Build history of the part. All positions in model axes, mm. Face numbers are marked on the shaded views. A direction names the side the tool comes from. Round coordinates to 2 decimals unless told otherwise and drop trailing zeros. Write each loop counter-clockwise with the first axis right and the second up, starting at its lowest first coordinate (ties: lowest second). Pieces come first, ordered by that corner, then holes.
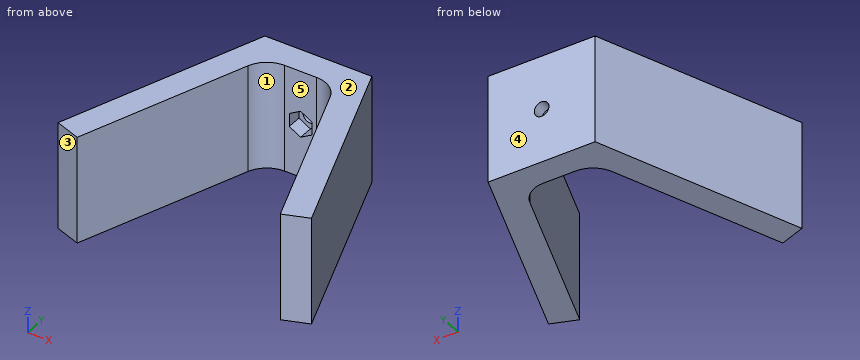
from build123d import *

# Parameters (mm, degrees)
F1_DEPTH = 40
F3_R     = 2.75
F4_DEPTH = 10
F5_R     = 2.75
F6_DEPTH = 5.5
F7_R     = 10


with BuildPart() as f1:
    # F0 (on Top) → F1 (new body)
    with BuildSketch(Plane.XY):
        Polygon((0, 0), (-20, 0), (-20, -10), (-12.9979246179, -10), (0, -10), align=None)
        Polygon((-20, -10), (-20, 0), (-47.3616114661, -75.1754096629), (-37.9646852582, -78.5956110961), (-12.9979246179, -10), align=None)
    extrude(amount=F1_DEPTH)

    # F2: F1 across plane


with BuildPart() as f1_1:
    add(f1.part)
    add(f1.part.mirror(Plane.YZ))

    # F3 (on face) → F4 (cut, through all)
    with BuildSketch(Plane.XZ.offset(10)):
        with Locations((0, 20)):
            Circle(F3_R)
    extrude(amount=-F4_DEPTH, mode=Mode.SUBTRACT)

    # F5 (on face) → F6 (cut)
    with BuildSketch(Plane.XZ.offset(10)):
        Polygon((4.25, 22.4537386441), (0, 24.9074772881), (-4.25, 22.4537386441), (-4.25, 17.5462613559), (0, 15.0925227119), (4.25, 17.5462613559), align=None)
        with Locations((0, 20)):
            Circle(F5_R, mode=Mode.SUBTRACT)
    extrude(amount=-F6_DEPTH, mode=Mode.SUBTRACT)

    # F7
    f7_edges = [f1_1.edges().sort_by_distance(p)[0] for p in [
        (-12.997925, -10, 20),
        (12.997925, -10, 20),
    ]]
    fillet(f7_edges, radius=F7_R)


solid = f1_1.part
1) Wall check: L1, parallel to Z at x = 0, y = -3.2; L2, parallel to X at y = -49, z = 5.5; L3, parallel to X at y = -30.5, z = 23. Give the ranges that are in metal, low to high.
Results:
L1: z = 0 to 17.25, 22.75 to 40
L2: x = -37.83 to -27.19, 27.19 to 37.83
L3: x = -31.1 to -20.46, 20.46 to 31.1
2) Slice it at B-B (z = 30.5). Write the cut outline in (x, y).
Results:
outline: (-47.36, -75.18) - (-37.96, -78.6) - (-15.39, -16.58) arc R10 cw to (-6, -10) - (6, -10) arc R10 cw to (15.39, -16.58) - (37.96, -78.6) - (47.36, -75.18) - (20, 0) - (-20, 0) - close
3) Pin check, flat tips, straight feed: pin 1 Ø1.5 at (x, z) = (2, 27) entering from -Y; pin 2 Ø10 at (y, z) = (-30.5, 26) entering from +X; pin 3 Ø4 at (y, z) = (-8, 20.5) entering from -X. Stop position of each tip, or through.
Results:
pin 1: stops at y = -10
pin 2: stops at x = 32.92
pin 3: stops at x = -23.64
4) Slice it at C-C (y = -12). Write the cut outline in (x, z).
Results:
outline: (-24.37, 0) - (-12, 0) - (-12, 40) - (-24.37, 40) - close; (12, 0) - (24.37, 0) - (24.37, 40) - (12, 40) - close
5) Mould opens along X. For the marked faces 1, 2 and 3 say: released by +X, released by -X, zero draft, split by the parting line, or undercut.
Results:
face 1: undercut
face 2: zero draft
face 3: released by -X
6) Slice it at A-A (z = 20). Write the cut outline in (x, y).
Results:
outline: (-47.36, -75.18) - (-37.96, -78.6) - (-15.39, -16.58) arc R10 cw to (-6, -10) - (-4.25, -10) - (-4.25, -4.5) - (-2.75, -4.5) - (-2.75, 0) - (-20, 0) - close; (2.75, -4.5) - (4.25, -4.5) - (4.25, -10) - (6, -10) arc R10 cw to (15.39, -16.58) - (37.96, -78.6) - (47.36, -75.18) - (20, 0) - (2.75, 0) - close
7) Slice it at D-D (y = -57.5). Write the cut outline in (x, z), plus the area to 3 significant figures.
Results:
outline: (-40.93, 0) - (-30.29, 0) - (-30.29, 40) - (-40.93, 40) - close; (30.29, 0) - (40.93, 0) - (40.93, 40) - (30.29, 40) - close
area: 851 mm2
8) Which spindle directions (+Z, -Z, +X, -X, +Y, -Y) get a long thin tool onto all of the face, cutting with end or side? Do the marked faces 4 and 5. Say none if no direction does.
Results:
face 4: +Z, -Z, +X, -X, +Y
face 5: +Z, -Z, -Y
